Geometry: see drawing. Coordinates: mm, zero at the bounding-box minimum. A direction names the side the tool comes from. Coordinates: 2 decimals unless noted, no trailing zeros. Loops run counter-clockwise (first coordinate to the right, second up) from the corner with the lowest first, then second, coordinate; pieces in that order, holes last.
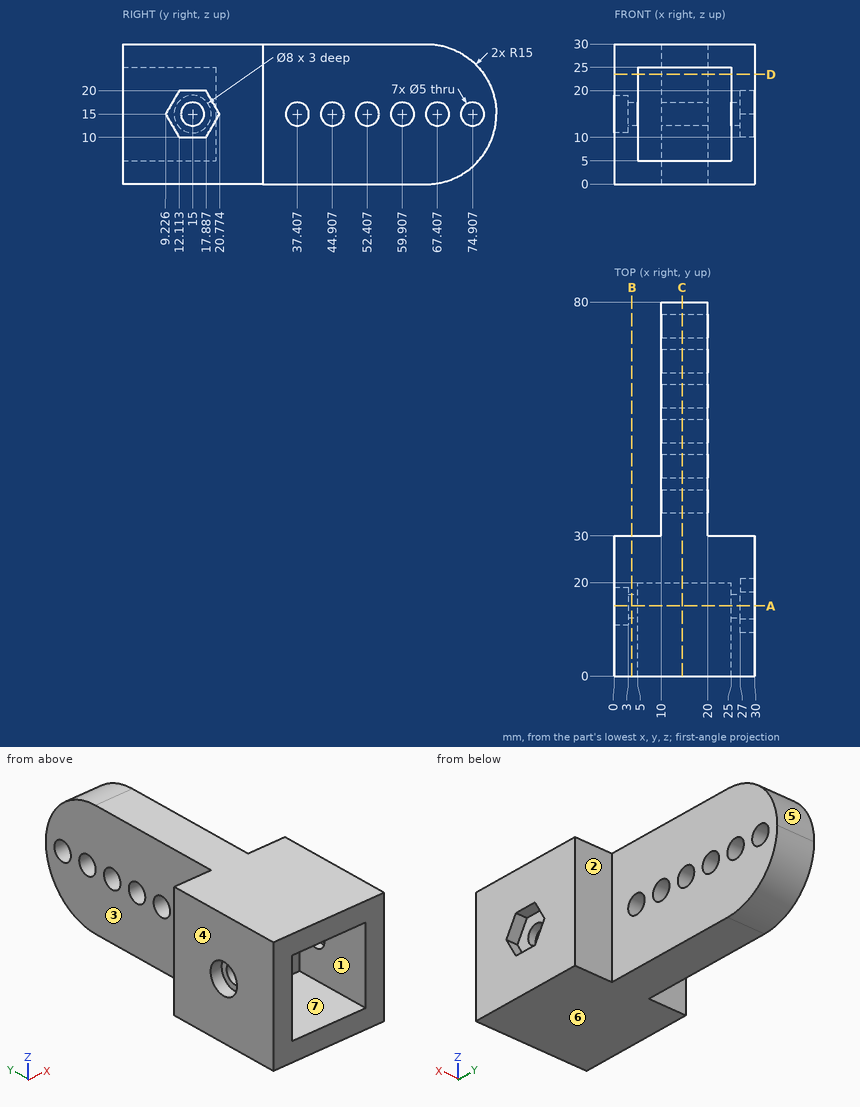
Item 1: Section query B-B (x = 3.75). Output: boundary loops of the cut face in (y, z).
Result:
outline: (0, 0) - (30, 0) - (30, 30) - (0, 30) - close; hole circle Ø5 at (15, 15)
Item 2: Line query: L1, parallel to X at y = 11, z = 22.5; L2, parallel to Y at x = 3.75, z = 15; L3, parallel to X at y = 41.5, z = 19. Output: solid intervals per line, ascending.
Result:
L1: x = 0 to 5, 25 to 30
L2: y = 0 to 12.5, 17.5 to 30
L3: x = 10 to 20
Item 3: Reachability of the marked faces 1, 2 and 3 from +Z, -Z, +X, -X, +Y, -Y: full face, straight path, thin tool, end or side. Return the list, or none.
Result:
face 1: -Y
face 2: +Z, -Z, +X, +Y
face 3: +Z, -Z, -X, +Y
Item 4: Mould query, pull axis Z, two halves, no side actions, for the marked faces 4, 5, 6 and 7. Classes: +Z half, -Z half, draft (parallel to the pull), parting line (faces both ways), or undercut.
Result:
face 4: draft
face 5: +Z half
face 6: -Z half
face 7: undercut
Item 5: Section query D-D (z = 23.5). Output: boundary loops of the cut face in (x, y).
Result:
outline: (0, 0) - (5, 0) - (5, 20) - (25, 20) - (25, 0) - (30, 0) - (30, 30) - (20, 30) - (20, 77.36) - (10, 77.36) - (10, 30) - (0, 30) - close
Item 6: Contact query for flat-ended pins moving along their axis: P1, Ø1.5, axis at x = 15.5, y = 67, coming from the -Z side; P2, Ø5, axis at y = 33.5, z = 15.5, coming from the -X side; P3, Ø1, axis at y = 58.5, z = 22.5, coming from the +X side. Output: stop coordinate, or through.
Result:
P1: stops at z = 0.05
P2: stops at x = 10
P3: stops at x = 20
Item 7: Section query A-A (y = 15). Output: boundary loops of the cut face in (x, z), then the cut area to 3 significant figures.
Result:
outline: (0, 0) - (30, 0) - (30, 10) - (27, 10) - (27, 12.5) - (25, 12.5) - (25, 5) - (5, 5) - (5, 12.5) - (3, 12.5) - (3, 11) - (0, 11) - close; (0, 19) - (3, 19) - (3, 17.5) - (5, 17.5) - (5, 25) - (25, 25) - (25, 17.5) - (27, 17.5) - (27, 20) - (30, 20) - (30, 30) - (0, 30) - close
area: 426 mm2
Item 8: Section query C-C (x = 14.5). Count the separate pieces of the cut face and the enclosed holes in it, then the cut area to 3 significant figures.
Result:
separate pieces: 1
enclosed holes: 6
area: 1,790 mm2
